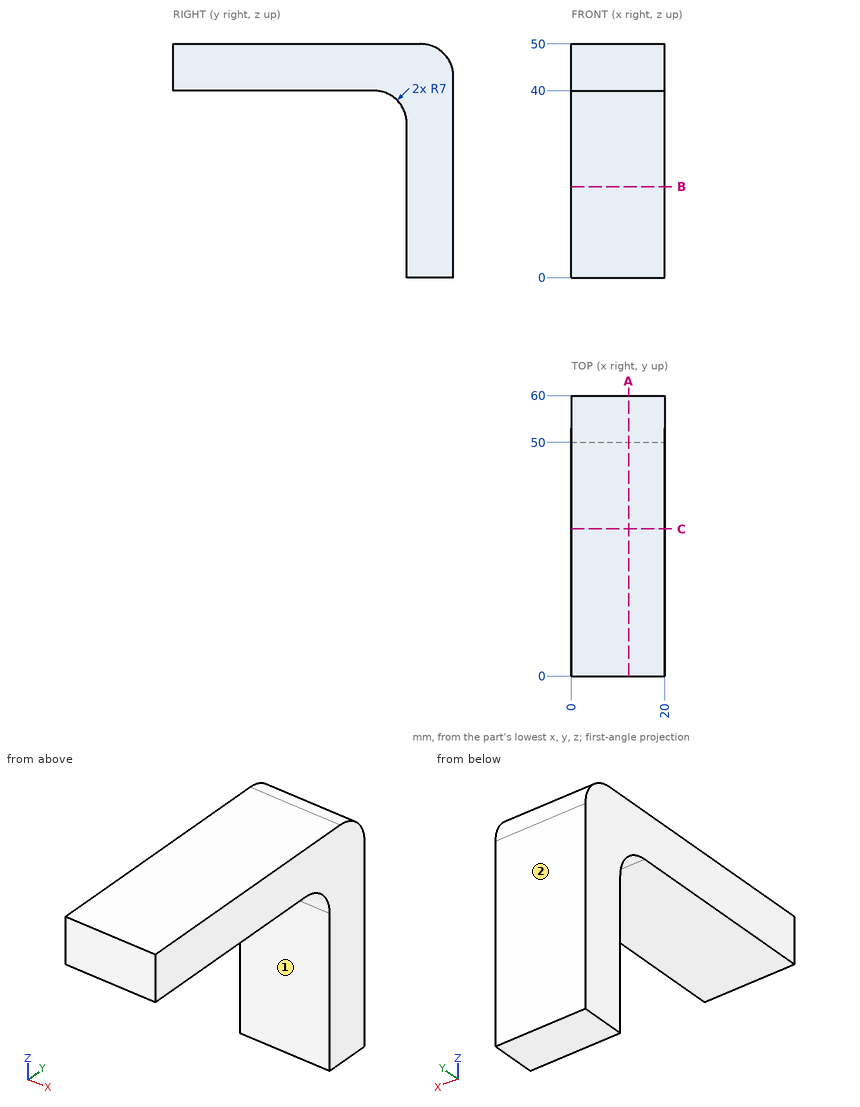
Source: three-view drawing plus pictorial views. Frame: mm from the lowest corner of the part. A direction names the side the tool comes from. Coordinates: 2 decimals unless noted, no trailing zeros. Loops run counter-clockwise (first coordinate to the right, second up) from the corner with the lowest first, then second, coordinate; pieces in that order, holes last. Notation, with made-up numbers: (-19.75, 51.25) -> (14.25, 51.25) arc R20 cw to (14.25, 82.25) -> close; hole circle Ø2 at (50.5, 8). An arc over 180 degrees is marked (long way). Write each question's results on one line, items separated by ' | '. Start each with the question number.
Q1. Section B-B, the plane z = 19.5. Return the cut outline in (x, y).
Q2. Section A-A, the plane x = 12.25. Return the cut outline in (y, z), plus the area to 3 significant figures.
Q3. Reachability of the marked faces 1 and 2 from +Z, -Z, +X, -X, +Y, -Y: full face, straight path, thin tool, end or side. Return the list, or none.
Q4. Section C-C, the plane y = 31.5. Return the cut outline in (x, z).
Q5. Pin query (flat end, axial travel): pin 1 (1.5 mm diameter, centred on x = 11, y = 27.5, fed in from -Z); pin 2 (3 mm diameter, centred on x = 5, z = 19, fed in from -Y); pin 3 (4 mm diameter, centred on y = 54, z = 45, fed in from -X); pin 4 (8 mm diameter, centred on y = 45.5, z = 12, fed in from +X). Return the tip coordinate at first contact, or that it passes through.
Q6. Ray query, line 1 (Y direction, x = 16.25, z = 25); line 2 (Z direction, x = 16.25, y = 43); line 3 (Z direction, x = 7, y = 46). Return the intervals inside material, ascending. Write a range as from..to.
Found:
1) outline: (0, 50) -> (20, 50) -> (20, 60) -> (0, 60) -> close
2) outline: (0, 40) -> (43, 40) arc R7 cw to (50, 33) -> (50, 0) -> (60, 0) -> (60, 43) arc R7 ccw to (53, 50) -> (0, 50) -> close | area: 1,000 mm2
3) face 1: -Z, +X, -X, -Y | face 2: +Z, -Z, +X, -X, +Y
4) outline: (0, 40) -> (20, 40) -> (20, 50) -> (0, 50) -> close
5) pin 1: z = 40 | pin 2: y = 50 | pin 3: x = 0 | pin 4: through
6) line 1: 50..60 | line 2: 40..50 | line 3: 39.32..50
